CAD build for the part. Positions are in the model's coordinates, mm. Face numbers are marked on the shaded views. Round coordinates to 2 decimals unless told otherwise and drop trailing zeros. Write each loop counter-clockwise with the first axis right and the second up, starting at its lowest first coordinate (ties: lowest second). Pieces come first, ordered by that corner, then holes. Notation, with made-up numbers: (3.25, 76.5) -> (48.25, 76.5) arc R18 ccw to (48.25, 104.5) -> close; hole circle Ø5 at (-8, -26). An arc over 180 degrees is marked (long way). Answer in a Markdown table with one row per item. Add a question column.
```python
from build123d import *

# Parameters (mm, degrees)
SKETCH1_R           = 1.25
BOSS_EXTRUDE1_DEPTH = 7
SKETCH2_R           = 1.2
CUT_EXTRUDE1_DEPTH  = 8


with BuildPart() as part:
    # Sketch1 → Boss-Extrude1 (new body)
    with BuildSketch(Plane(origin=(0, 0, 0), x_dir=(1, 0, 0), z_dir=(0, 1, 0))):
        with BuildLine():
            Line((-0.481545064, 2.70751073), (-8.5, 2))
            ThreePointArc((-8.5, 2), (-10.5, 0), (-8.5, -2))
            Line((-8.5, -2), (-0.481545064, -2.70751073))
            Line((-0.481545064, -2.70751073), (0, -2.75))
            ThreePointArc((0, -2.75), (2.75, 0), (0, 2.75))
            Line((0, 2.75), (-0.481545064, 2.70751073))
        make_face()
        Circle(SKETCH1_R, mode=Mode.SUBTRACT)
    extrude(amount=BOSS_EXTRUDE1_DEPTH)

    # Sketch2 → Cut-Extrude1 (cut)
    with BuildSketch(Plane.ZY.offset(10.5)):
        with Locations((0, 3.5)):
            Circle(SKETCH2_R)
    extrude(amount=-CUT_EXTRUDE1_DEPTH, mode=Mode.SUBTRACT)


solid = part.part
```
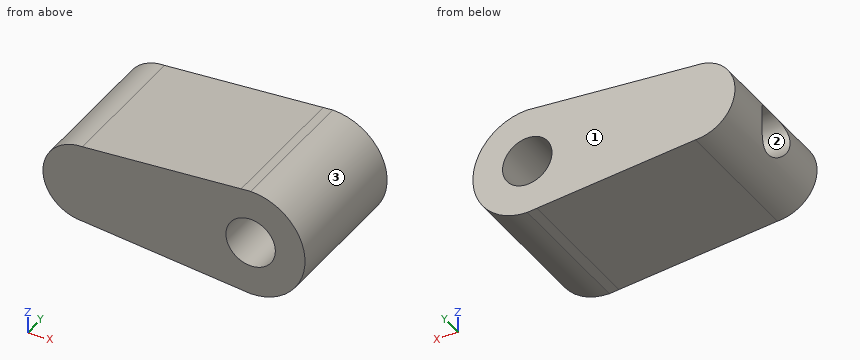
Item 1: Saw through at D-D on x = -2.75. Give the cut face in (y, z), then the cut area to 3 significant figures.
Item 2: Saw through at A-A on z = 0. Give the cut face in (x, y).
Item 3: Saw through at B-B on y = 5.75. Give the cut face in (x, z), then the cut area to 3 significant figures.
Item 4: Two-plate mould, pull along Y, no slides. Class the marked faces 1, 2 and 3: +Y half, -Y half, draft (parallel to the pull), parting line (faces both ways), or undercut.
Item 5: Saw through at C-C on x = 1. Give the cut face in (y, z), then the cut area to 3 significant figures.
Item 6: Drill centre lines: probe 1 along Y at (x, z) = (-5.5, 0); probe 2 along Z at (x, y) = (0, 1.75); probe 3 along X at (y, z) = (5, 0). Where is each one in solid material? Low to high.
Item 7: Pin check, flat tips, straight feed: pin 1 (1.2 mm diameter, centred on y = 3.5, z = 0, fed in from -X); pin 2 (2 mm diameter, centred on y = 1.5, z = -2, fed in from +X); pin 3 (2 mm diameter, centred on x = -2, y = 1.5, fed in from +Z); pin 4 (3 mm diameter, centred on x = -6, z = -1.5, fed in from -Y). Stop position of each tip, or through.
Recorded:
| question | item | result |
|---|---|---|
| 1 | outline | (0, -2.51) -> (7, -2.51) -> (7, 2.51) -> (0, 2.51) -> close; hole circle Ø2.4 at (3.5, 0) |
| 1 | area | 30.6 mm2 |
| 2 | outline | (-10.5, 0) -> (-1.25, 0) -> (-1.25, 7) -> (-10.5, 7) -> (-10.5, 4.7) -> (-2.5, 4.7) -> (-2.5, 2.3) -> (-10.5, 2.3) -> close; (1.25, 0) -> (2.75, 0) -> (2.75, 7) -> (1.25, 7) -> close |
| 3 | outline | (-8.5, -2) -> (0, -2.75) arc R2.75 ccw to (0, 2.75) -> (-8.5, 2) arc R2 ccw to start; hole circle Ø2.5 at (0, 0) |
| 3 | area | 53.6 mm2 |
| 4 | face 1 | +Y half |
| 4 | face 2 | undercut |
| 4 | face 3 | draft |
| 5 | outline | (0, -2.56) -> (7, -2.56) -> (7, -0.75) -> (0, -0.75) -> close; (0, 0.75) -> (7, 0.75) -> (7, 2.56) -> (0, 2.56) -> close |
| 5 | area | 25.4 mm2 |
| 6 | probe 1 | 0 to 2.3, 4.7 to 7 |
| 6 | probe 2 | -2.75 to -1.25, 1.25 to 2.75 |
| 6 | probe 3 | -10.5 to -1.25, 1.25 to 2.75 |
| 7 | pin 1 | x = -2.5 |
| 7 | pin 2 | x = 2.56 |
| 7 | pin 3 | z = 2.66 |
| 7 | pin 4 | y = 0 |
